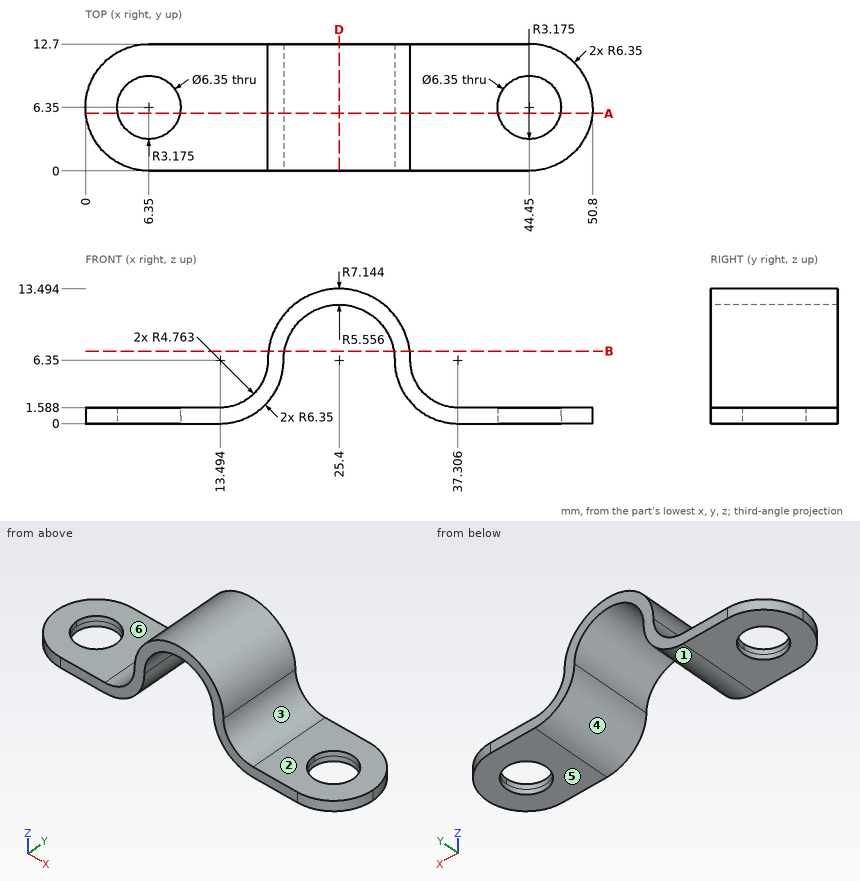
Design review of the part shown in the three views and the two pictorial views. Dimensions are in mm from the part's minimum x, y and z. A direction names the side the tool comes from. Round coordinates to 2 decimals unless told otherwise and drop trailing zeros. Loops run counter-clockwise (first coordinate to the right, second up) from the corner with the lowest first, then second, coordinate; pieces in that order, holes last. Notation, with made-up numbers: (-22.75, 10) - (-9.75, 10) arc R27 cw to (-9.75, 30) - close; hole circle Ø9 at (-27, -20.75). An arc over 180 degrees is marked (long way). Write each question's results on one line, items separated by ' | '. Start each with the question number.
Q1. Take a section at D-D on x = 25.4. Give the boundary of the cut face in (y, z).
Q2. Insertion check: P1, Ø7.5, axis at x = 44.45, y = 6.35, coming from the +Z side; P2, Ø1, axis at y = 4.5, z = 5.5, coming from the +X side. Each pin has a flat end and moves straight along its axis. Give the tip position at first contact, or say it passes through.
Q3. Tool access review of the marked faces 4, 5 and 6: name each direction out of +Z, -Z, +X, -X, +Y, -Y from which nothing blocks a thin tool from reaching the whole face with its end or side.
Q4. Take a section at A-A on y = 5.75. Give the number of separate pieces and of enclosed holes in the cut face.
Q5. Wall thickness on line 1 along Y through (x, z) = (6.35, 0.3) (1 decimal); line 2 along Z through (x, y) = (12.5, 4.25); line 3 along Z through (x, y) = (25.5, 6) (1 decimal): over which ranges is each line inside the solid? List them lowest first. Write a range as [from, to].
Q6. Draft analysis for pull direction X (two halves, no side actions). For the marked faces 1, 2 and 3, state which applies: pulls with the +X half, pulls with the -X half, needs draft (parallel to the pull), parting line crosses it, or undercut.
Q7. Take a section at B-B on z = 7.25. Give the boundary of the cut face in (x, y).
Data:
1) outline: (0, 11.91) - (12.7, 11.91) - (12.7, 13.49) - (0, 13.49) - close
2) P1: stops at z = 1.59 | P2: stops at x = 32.74
3) face 4: -Z, +Y, -Y | face 5: -Z, +X, -X, +Y, -Y | face 6: +Z, -X, +Y, -Y
4) separate pieces: 3 | enclosed holes: 0
5) line 1: y = [0, 3.2], [9.5, 12.7] | line 2: z = [0, 1.59] | line 3: z = [11.9, 13.5]
6) face 1: undercut | face 2: needs draft | face 3: pulls with the +X half
7) outline: (18.31, 0) - (19.92, 0) - (19.92, 12.7) - (18.31, 12.7) - close; (30.88, 0) - (32.49, 0) - (32.49, 12.7) - (30.88, 12.7) - close
